The figure shows three views and two pictorial views of one solid part (mm, origin at its lowest corner). Answer the questions. Give positions to 0.01 mm unless a question says otherwise; leave off trailing zeros. Write each loop counter-clockwise with the first axis right and the second up, starting at its lowest first coordinate (ties: lowest second). Pieces come first, ordered by that corner, then holes. Notation, with made-up numbers: (45, -28.5) -> (88, -28.5) arc R26 ccw to (88, -7.5) -> close; hole circle Ø6 at (-32, 1). An arc over 180 degrees is marked (long way). Use a Markdown table: item, result.
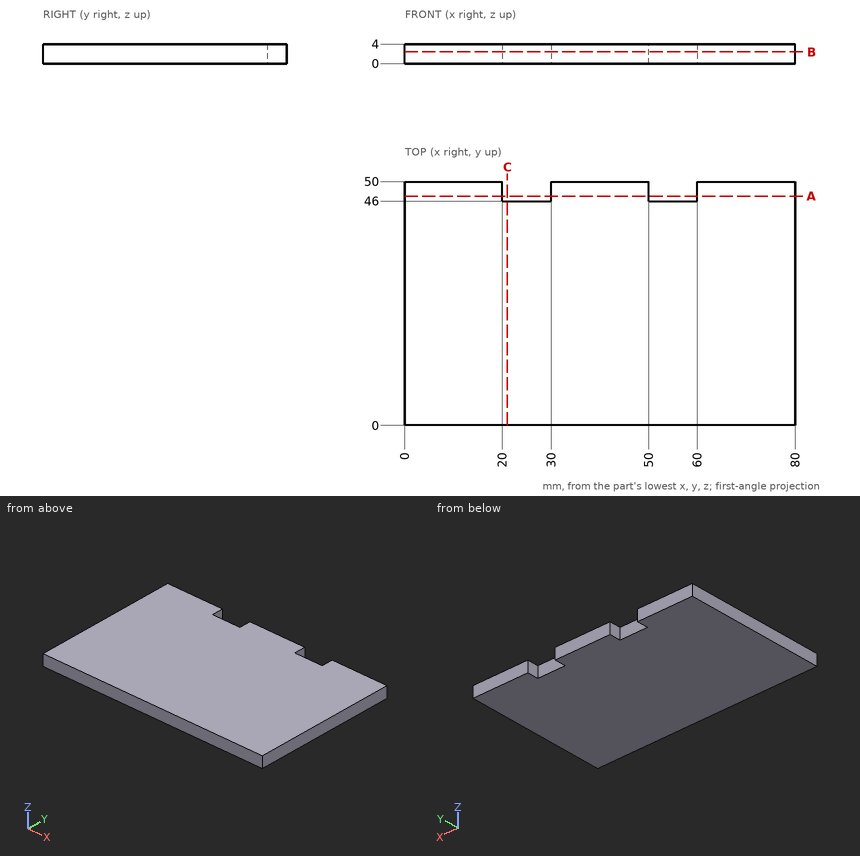
Item 1: A straight line is drawn through the part: line 1 along Y through (x, z) = (27.5, 3.1). Find the intervals that lie inside material, in ascending order. Write a range as [from, to].
Return value:
| item | result |
|---|---|
| line 1 | [0, 46] |
Item 2: A cutting plane is placed at A-A (y = 47). Give the vertices of the cut face in (x, z).
Return value:
| item | result |
|---|---|
| outline | (0, 0) -> (20, 0) -> (20, 4) -> (0, 4) -> close; (30, 0) -> (50, 0) -> (50, 4) -> (30, 4) -> close; (60, 0) -> (80, 0) -> (80, 4) -> (60, 4) -> close |
Item 3: A cutting plane is placed at B-B (z = 2.4). Give the vertices of the cut face in (x, y), then the cut area to 3 significant figures.
Return value:
| item | result |
|---|---|
| outline | (0, 0) -> (80, 0) -> (80, 50) -> (60, 50) -> (60, 46) -> (50, 46) -> (50, 50) -> (30, 50) -> (30, 46) -> (20, 46) -> (20, 50) -> (0, 50) -> close |
| area | 3,920 mm^2 |
Item 4: A cutting plane is placed at C-C (x = 21). Give the vertices of the cut face in (y, z).
Return value:
| item | result |
|---|---|
| outline | (0, 0) -> (46, 0) -> (46, 4) -> (0, 4) -> close |
